For this review, use the dimensioned drawing (mm, ordinates from the lowest corner) and the shaded views. Round coordinates to 2 decimals unless told otherwise and drop trailing zeros. Loops run counter-clockwise (first coordinate to the right, second up) from the corner with the lowest first, then second, coordinate; pieces in that order, holes last. Notation, with made-up numbers: (15.25, 27.5) -> (48.25, 27.5) arc R16 ccw to (48.25, 58.5) -> close; hole circle Ø1 at (32.5, -39.75). An arc over 180 degrees is marked (long way). Answer as CSV lines item,"result". Start each with the question number.
(1) For P1, Ø4, axis at x = 15.5, z = 10, coming from the -Y side; P2, Ø1.3, axis at y = 2.5, z = 26.5, coming from the +X side; P3, Ø3, axis at x = 22.5, z = 25.5, coming from the -Y side, all flat-tipped, find the tip position at first contact; note any pin that passes through.
(2) Take a section at C-C, the plane y = 0.9. Write out the cut boundary in (x, z).
(3) Take a section at A-A, the plane z = 10. Write out the cut boundary in (x, y).
(4) Take a section at B-B, the plane x = 15.5. Write out the cut boundary in (y, z).
(5) Take a section at D-D, the plane x = 3.5. Write out the cut boundary in (y, z), and give its area (3 significant figures).
(6) To check wall thickness, follow line 1 (Z direction, x = 15.5, y = 1.25); line 2 (X direction, y = 1.75, z = 20); line 3 (X direction, y = 1.6, z = 10.5) (1 decimal). State the ranges of each line that lie inside material, in increasing order. Write a range as from..to.
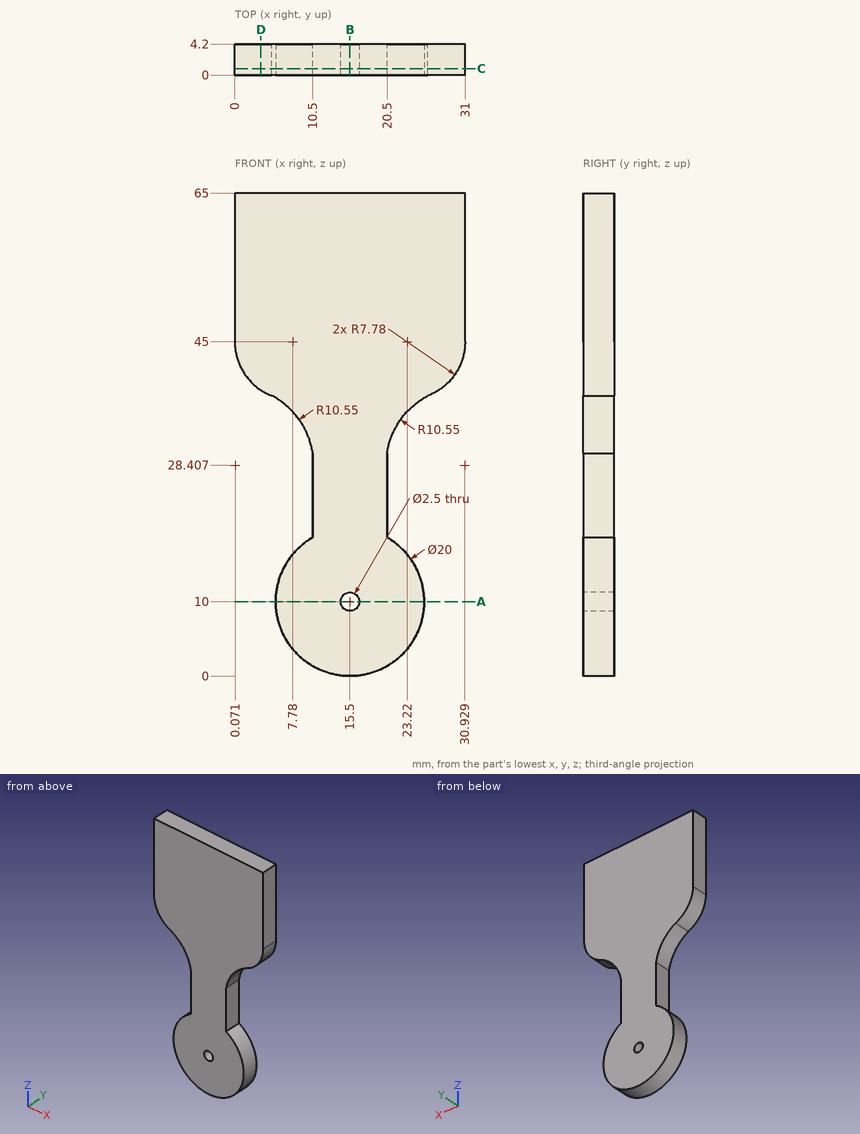
The answers:
1,P1,"y = 0"
1,P2,"x = 20.5"
1,P3,"through"
2,outline,"(0, 45) arc R7.78 ccw to (5, 37.73) arc R10.55 cw to (10.5, 30) -> (10.5, 18.66) arc R10 ccw (long way) to (20.5, 18.66) -> (20.5, 30) arc R10.55 cw to (26, 37.73) arc R7.78 ccw to (31, 45) -> (31, 65) -> (0, 65) -> close; hole circle Ø2.5 at (15.5, 10)"
3,outline,"(5.5, 0) -> (14.25, 0) -> (14.25, 4.2) -> (5.5, 4.2) -> close; (16.75, 0) -> (25.5, 0) -> (25.5, 4.2) -> (16.75, 4.2) -> close"
4,outline,"(0, 0) -> (4.2, 0) -> (4.2, 8.75) -> (0, 8.75) -> close; (0, 11.25) -> (4.2, 11.25) -> (4.2, 65) -> (0, 65) -> close"
5,outline,"(0, 38.5) -> (4.2, 38.5) -> (4.2, 65) -> (0, 65) -> close"
5,area,"111 mm²"
6,line 1,"0..8.75, 11.25..65"
6,line 2,"10.5..20.5"
6,line 3,"5.5..14.4, 16.6..25.5"
